For this review, take the finished solid that the model builds, in its own axes (mm). Face numbers are marked on the shaded views. A direction names the side the tool comes from. Coordinates: 2 decimals unless noted, no trailing zeros. Loops run counter-clockwise (first coordinate to the right, second up) from the corner with the lowest first, then second, coordinate; pieces in that order, holes last.
1. Mouldability with a two-part tool opening along X and no side actions: class the marked faces 1, 2 and 3 as pulls with the +X half, pulls with the -X half, needs draft (parallel to the pull), parting line crosses it, or undercut.
2. To check wall thickness, follow probe 1 along Z at (x, y) = (-12, -8.75); probe 2 along Y at (x, z) = (0, 9.5); probe 3 along X at (y, z) = (1.75, -11). State the ranges of each line that lie inside material, in increasing order.
3. Take a section at C-C, the plane y = 0. Count the separate pieces of the cut face and the enclosed holes in it, then the cut area to 3 significant figures.
4. Machinability: for the marked faces 4, 5 and 6, which of the approach directions +Z, -Z, +X, -X, +Y, -Y give a long, thin tool a straight path to every point of the face, cutting with its end or side? Answer none if there is none.
5. Take a section at D-D, the plane x = 0. State the section outline as (y, z) points, then the cut area to 3 significant figures.
6. Take a section at B-B, the plane x = 18.5. State the section outline as (y, z) points.
7. Clearance check with flat-ended pins moving along their axes: P1, Ø12.5, axis at x = -16.5, y = -2, coming from the -Z side; P2, Ø8, axis at x = -8.5, z = -8, coming from the -Y side; P3, Ø12, axis at x = 10, z = -25, coming from the +Y side. State where each tip first meets the part, or that it passes through.
8. Take a section at A-A, the plane z = -15.5. State the section outline as (x, y) points, then the cut area to 3 significant figures.
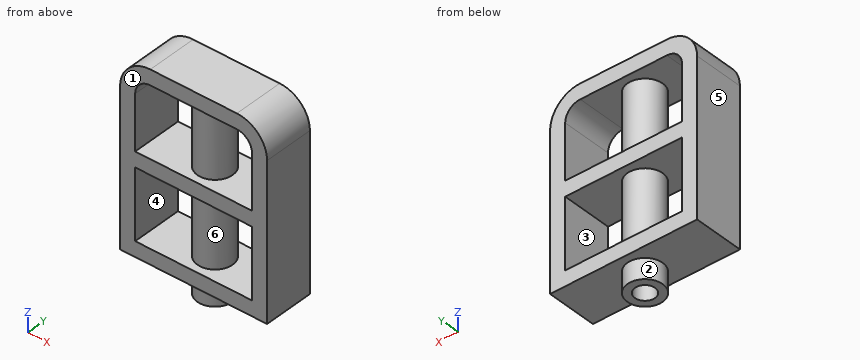
```python
from build123d import *

# Parameters (mm, degrees)
CROQUIS1_W                   = 58
CROQUIS1_H                   = 34.75
SALIENTE_EXTRUIR1_DEPTH      = 12.5
CROQUIS2_R                   = 8.75
SALIENTE_EXTRUIR2_DEPTH      = 10
SALIENTE_EXTRUIR2_DEPTH_BACK = 84.5
CROQUIS3_R                   = 5
CORTAR_EXTRUIR1_DEPTH        = 94.5


with BuildPart() as part:
    # Croquis1 → Saliente-Extruir1 (new body, symmetric)
    with BuildSketch(Plane(origin=(0, 0, 0), x_dir=(1, 0, 0), z_dir=(0, 1, 0))):
        with BuildLine():
            Line((21.5, -46), (-21.5, -46))
            ThreePointArc((-21.5, -46), (-32.106601718, -41.606601718), (-36.5, -31))
            Line((-36.5, -31), (-36.5, 46))
            Line((-36.5, 46), (36.5, 46))
            Line((36.5, 46), (36.5, -31))
            ThreePointArc((36.5, -31), (32.106601718, -41.606601718), (21.5, -46))
        make_face()
        with BuildLine():
            Line((-29, -31), (-29, -3.75))
            Line((-29, -3.75), (29, -3.75))
            Line((29, -3.75), (29, -31))
            ThreePointArc((29, -31), (26.803300859, -36.303300859), (21.5, -38.5))
            Line((21.5, -38.5), (-21.5, -38.5))
            ThreePointArc((-21.5, -38.5), (-26.803300859, -36.303300859), (-29, -31))
        make_face(mode=Mode.SUBTRACT)
        with Locations((0, 21.125)):
            Rectangle(CROQUIS1_W, CROQUIS1_H, mode=Mode.SUBTRACT)
    extrude(amount=SALIENTE_EXTRUIR1_DEPTH, both=True)

    # Croquis2 → Saliente-Extruir2 (add, two sides)
    with BuildSketch(Plane(origin=(0, 0, -46), x_dir=(-1, 0, 0), z_dir=(0, 0, -1))) as saliente_extruir2_sk:
        Circle(CROQUIS2_R)
    extrude(amount=SALIENTE_EXTRUIR2_DEPTH)
    extrude(saliente_extruir2_sk.sketch, amount=-SALIENTE_EXTRUIR2_DEPTH_BACK)

    # Croquis3 → Cortar-Extruir1 (cut)
    with BuildSketch(Plane(origin=(0, 0, -56), x_dir=(-1, 0, 0), z_dir=(0, 0, -1))):
        Circle(CROQUIS3_R)
    extrude(amount=-CORTAR_EXTRUIR1_DEPTH, mode=Mode.SUBTRACT)


solid = part.part
```
Results list:
1. face 1: needs draft
1. face 2: parting line crosses it
1. face 3: undercut
2. probe 1: z = -46 to -38.5, -3.75 to 3.75, 38.5 to 46
2. probe 2: y = -8.75 to -5, 5 to 8.75
2. probe 3: x = -36.5 to -29, -8.57 to -4.68, 4.68 to 8.57, 29 to 36.5
3. separate pieces: 1
3. enclosed holes: 4
3. area: 3,060 mm2
4. face 4: +Y, -Y
4. face 5: +Z, -Z, -X, +Y, -Y
4. face 6: none
5. outline: (-12.5, -46) - (-8.75, -46) - (-8.75, -56) - (-5, -56) - (-5, 38.5) - (5, 38.5) - (5, -56) - (8.75, -56) - (8.75, -46) - (12.5, -46) - (12.5, -38.5) - (8.75, -38.5) - (8.75, -3.75) - (12.5, -3.75) - (12.5, 3.75) - (8.75, 3.75) - (8.75, 38.5) - (12.5, 38.5) - (12.5, 46) - (-12.5, 46) - (-12.5, 38.5) - (-8.75, 38.5) - (-8.75, 3.75) - (-12.5, 3.75) - (-12.5, -3.75) - (-8.75, -3.75) - (-8.75, -38.5) - (-12.5, -38.5) - close
5. area: 1,010 mm2
6. outline: (-12.5, -46) - (12.5, -46) - (12.5, -38.5) - (-12.5, -38.5) - close; (-12.5, -3.75) - (12.5, -3.75) - (12.5, 3.75) - (-12.5, 3.75) - close; (-12.5, 38.5) - (12.5, 38.5) - (12.5, 46) - (-12.5, 46) - close
7. P1: stops at z = -46
7. P2: stops at y = -7.5
7. P3: stops at y = 7.78
8. outline: (-36.5, -12.5) - (-29, -12.5) - (-29, 12.5) - (-36.5, 12.5) - close; circle Ø17.5 at (0, 0); (29, -12.5) - (36.5, -12.5) - (36.5, 12.5) - (29, 12.5) - close; hole circle Ø10 at (0, 0)
8. area: 537 mm2
